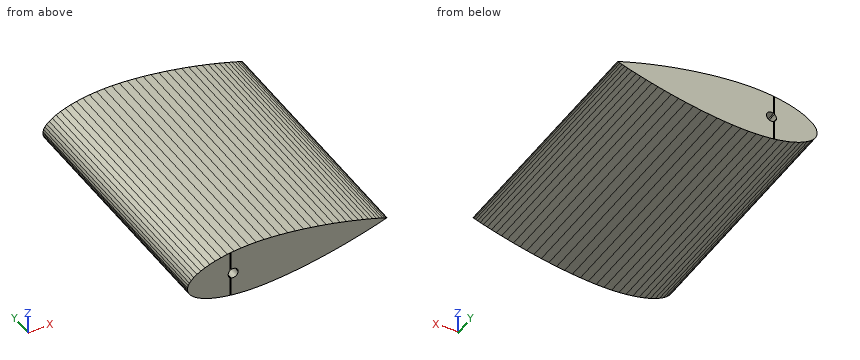
from build123d import *

# Parameters (mm, degrees)
F1_DEPTH = 1000
F3_DEPTH = 1000
F4_DEPTH = 1100


# Not quite as in the source:
# - a feature names something its author has since deleted; it is built from what else it names


with BuildPart() as f1:
    # F0 (on Front) → F1 (new body)
    with BuildSketch(Plane.XZ):
        Polygon((398.8592052974, -22.0067325898), (399.1788252872, -21.8985260996), (398.86, -21.788), (395.252, -20.532), (389.268, -18.468), (380.924, -15.636), (370.284, -12.092), (357.388, -7.884), (342.308, -3.092), (325.124, 2.196), (305.94, 7.9), (284.86, 13.924), (261.996, 20.188), (237.476, 26.58), (211.46, 33.028), (184.092, 39.412), (155.54, 45.66), (125.964, 51.676), (95.556, 57.364), (64.508, 62.644), (32.996, 67.412), (1.236, 71.604), (-30.58, 75.124), (-62.236, 77.908), (-93.804, 79.86), (-125.172, 80.74), (-155.748, 80.484), (-185.332, 79.076), (-213.692, 76.532), (-240.636, 72.9), (-265.956, 68.236), (-289.484, 62.612), (-311.052, 56.124), (-330.516, 48.892), (-347.748, 41.02), (-362.66, 32.636), (-375.156, 23.868), (-385.18, 14.828), (-392.684, 5.62), (-397.644, -3.66), (-400.06, -12.948), (-399.9816032326, -18.9950039949), (-400.1039374883, -25.0412786908), (-397.7554909925, -34.3465889519), (-392.863053528, -43.6623849811), (-385.4261600494, -52.9246684677), (-375.4681123548, -62.0372675544), (-363.0361534783, -70.8958362025), (-348.1854681119, -79.3879704541), (-331.0111236302, -87.3849761202), (-311.6001876192, -94.7582171427), (-290.0799010007, -101.4027661761), (-266.5933880129, -107.1975800363), (-241.3079466524, -112.0454405133), (-214.3910493078, -115.8731287637), (-186.0502835732, -118.6231348681), (-156.4772955956, -120.2460649573), (-125.9039629887, -120.7242336641), (-94.530396734, -120.0721872989), (-62.949046248, -118.3496225018), (-31.2736524944, -115.7957191071), (0.567085058, -112.5069977565), (32.356707066, -108.5458872321), (63.9025210304, -104.006989863), (94.988067608, -98.9527344313), (125.4365957465, -93.4858393163), (155.0555292079, -87.6849072697), (183.6521754929, -81.6445406207), (211.0658412572, -75.4595742212), (237.1280077599, -69.2007854261), (261.6938068426, -62.9871247152), (284.602719553, -56.8894275739), (305.7259354409, -51.0187609546), (324.9508761562, -45.4543089157), (342.1728468763, -40.2913132239), (357.2872690402, -35.6090160683), (370.2135053222, -31.494833819), (380.8789763165, -28.0282411878), (389.2433342948, -25.256946254), (395.2421740321, -23.2364824938), align=None)
    extrude(amount=F1_DEPTH)

    # F2 (on face) → F3 (cut)
    with BuildSketch(Plane.XZ.offset(1000)):
        with BuildLine():
            ThreePointArc((-229.6033561446, -3.6511614936), (-235.4817946773, -10.6760485755), (-237.6118033553, -19.5849284785))
            Line((-237.6118033553, -19.5849284785), (-197.6120673578, -19.7302561417))
            ThreePointArc((-197.6120673578, -19.7302561417), (-206.6231942764, -2.9468900665), (-225.6033561446, -1.3235476449))
            Line((-225.6033561446, -1.3235476449), (-225.6033561446, 73.9173274625))
            Line((-225.6033561446, 73.9173274625), (-229.6033561446, 73.3781350635))
            Line((-229.6033561446, 73.3781350635), (-229.6033561446, -3.6511614936))
        make_face()
        with BuildLine():
            Line((-197.6120673578, -19.7302561417), (-237.6118033553, -19.5849284785))
            ThreePointArc((-237.6118033553, -19.5849284785), (-235.5465858175, -28.5090505427), (-229.7193476609, -35.5764668712))
            ThreePointArc((-229.7193476609, -35.5764668712), (-227.7962509426, -36.8703700071), (-225.736366484, -37.9330846114))
            ThreePointArc((-225.736366484, -37.9330846114), (-206.744909945, -36.4477012646), (-197.6120673578, -19.7302561417))
        make_face()
        with BuildLine():
            ThreePointArc((-225.736366484, -37.9330846114), (-227.7962509426, -36.8703700071), (-229.7193476609, -35.5764668712))
            Line((-229.7193476609, -35.5764668712), (-230.2790683503, -112.6037298424))
            Line((-230.2790683503, -112.6037298424), (-226.2830919036, -113.1719733475))
            Line((-226.2830919036, -113.1719733475), (-225.736366484, -37.9330846114))
        make_face()
    extrude(amount=-F3_DEPTH, mode=Mode.SUBTRACT)

    # F2 (on face) → F4 (cut)
    with BuildSketch(Plane.XZ.offset(1000)):
        with BuildLine():
            ThreePointArc((-229.6033561446, -3.6511614936), (-235.4817946773, -10.6760485755), (-237.6118033553, -19.5849284785))
            Line((-237.6118033553, -19.5849284785), (-197.6120673578, -19.7302561417))
            ThreePointArc((-197.6120673578, -19.7302561417), (-206.6231942764, -2.9468900665), (-225.6033561446, -1.3235476449))
            Line((-225.6033561446, -1.3235476449), (-225.6033561446, 73.9173274625))
            Line((-225.6033561446, 73.9173274625), (-229.6033561446, 73.3781350635))
            Line((-229.6033561446, 73.3781350635), (-229.6033561446, -3.6511614936))
        make_face()
        with BuildLine():
            Line((-197.6120673578, -19.7302561417), (-237.6118033553, -19.5849284785))
            ThreePointArc((-237.6118033553, -19.5849284785), (-235.5465858175, -28.5090505427), (-229.7193476609, -35.5764668712))
            ThreePointArc((-229.7193476609, -35.5764668712), (-227.7962509426, -36.8703700071), (-225.736366484, -37.9330846114))
            ThreePointArc((-225.736366484, -37.9330846114), (-206.744909945, -36.4477012646), (-197.6120673578, -19.7302561417))
        make_face()
        with BuildLine():
            ThreePointArc((-225.736366484, -37.9330846114), (-227.7962509426, -36.8703700071), (-229.7193476609, -35.5764668712))
            Line((-229.7193476609, -35.5764668712), (-230.2790683503, -112.6037298424))
            Line((-230.2790683503, -112.6037298424), (-226.2830919036, -113.1719733475))
            Line((-226.2830919036, -113.1719733475), (-225.736366484, -37.9330846114))
        make_face()
    extrude(amount=-F4_DEPTH, mode=Mode.SUBTRACT)


solid = f1.part
Geometry: final body of the model. Coordinates: model frame, mm. Coordinates: 2 decimals unless noted, no trailing zeros. Write each loop counter-clockwise with the first axis right and the second up, starting at its lowest first coordinate (ties: lowest second). Pieces come first, ordered by that corner, then holes. Notation, with made-up numbers: (76.25, 17.5) - (125.25, 17.5) arc R7 ccw to (125.25, 27.5) - close; hole circle Ø4 at (3, -13.5). An arc over 180 degrees is marked (long way). Return JSON: item names as keys, results as strings.
Item 1: Pin query (flat end, axial travel): pin 1 Ø10 at (y, z) = (-764.5, 22.5) entering from -X; pin 2 Ø10 at (x, y) = (84.5, -203) entering from -Z; pin 3 Ø1.5 at (x, z) = (-301, -74) entering from +Y; pin 4 Ø8 at (x, y) = (-304, -771) entering from -Z. Return the tip coordinate at first contact, or that it passes through.
Completed:
{"pin 1": "stops at x = -382.22", "pin 2": "stops at z = -101.47", "pin 3": "stops at y = 0", "pin 4": "stops at z = -98.34"}
Item 2: Section query A-A (x = 250). Output: boundary loops of the cut face in (y, z), and give its area (3 significant figures).
Completed:
{"outline": "(-1000, -65.94) - (0, -65.94) - (0, 23.32) - (-1000, 23.32) - close", "area": "89,300 mm2"}
Item 3: Line query: L1, parallel to Z at x = -64.5, y = -476; L2, parallel to Z at x = -341, y = -305.5. Output: solid intervals per line, ascending.
Completed:
{"L1": "z = -118.43 to 78.05", "L2": "z = -82.73 to 44.1"}
Item 4: Section query B-B (x = 84). Output: boundary loops of the cut face in (y, z), and give its area (3 significant figures).
Completed:
{"outline": "(-1000, -100.74) - (0, -100.74) - (0, 59.33) - (-1000, 59.33) - close", "area": "160,000 mm2"}
